Autodesk Inventor part; units mm, degrees
ref_plane "YZ Plane" through (0, 0, 0) normal (1, 0, 0) x (0, 1, 0)
ref_plane "XZ Plane" through (0, 0, 0) normal (0, 1, 0) x (-1, 0, 0)
ref_plane "XY Plane" through (0, 0, 0) normal (0, 0, 1) x (1, 0, 0)
sketch "Sketch7" plane through (0, 0, 0) normal (0, 1, 0) x (-1, 0, 0)
  line L0 (93.98, -93.98) -> (0, -93.98)
  line L1 (0, -87.376) -> (0, -6.604)
  circle A0 centre (101.4857, 19.3548) radius 1.85
  circle A1 centre (101.4857, 19.3548) radius 1.85
  circle A2 centre (-7.5057, 19.3548) radius 1.85
  circle A3 centre (-7.5057, 19.3548) radius 1.85
  circle A4 centre (-7.5057, -113.3348) radius 1.85
  circle A5 centre (101.4857, -113.3348) radius 1.85
  circle A6 centre (101.4857, -113.3348) radius 1.85
  arc A7 (104.7877, 19.3548) -> (98.1837, 19.3548) centre (101.4857, 19.3548) ccw
  arc A8 (-4.2037, 19.3548) -> (-10.8077, 19.3548) centre (-7.5057, 19.3548) ccw
  arc A9 (-10.8077, -113.3348) -> (-4.2037, -113.3348) centre (-7.5057, -113.3348) ccw
  arc A10 (98.1837, -113.3348) -> (104.7877, -113.3348) centre (101.4857, -113.3348) ccw
  line L2 (98.1837, 19.3548) -> (98.1837, 0)
  line L3 (98.1837, 0) -> (93.98, 0)
  line L4 (104.7877, 19.3548) -> (104.7877, 0)
  line L5 (104.7877, 0) -> (104.7877, -6.604)
  line L6 (104.7877, -6.604) -> (93.98, -6.604)
  arc A11 (98.1837, -113.3348) -> (104.7877, -113.3348) centre (101.4857, -113.3348) ccw
  line L7 (98.1837, -113.3348) -> (98.1837, -93.98)
  line L8 (98.1837, -93.98) -> (93.98, -93.98)
  line L9 (104.7877, -113.3348) -> (104.7877, -93.98)
  line L10 (104.7877, -93.98) -> (104.7877, -87.376)
  line L11 (104.7877, -87.376) -> (93.98, -87.376)
  arc A12 (-4.2037, 19.3548) -> (-10.8077, 19.3548) centre (-7.5057, 19.3548) ccw
  line L12 (-4.2037, 19.3548) -> (-4.2037, 0)
  line L13 (-4.2037, 0) -> (0, 0)
  line L14 (-10.8077, 19.3548) -> (-10.8077, 0)
  line L15 (-10.8077, 0) -> (-10.8077, -6.604)
  line L16 (-10.8077, -6.604) -> (0, -6.604)
  arc A13 (-10.8077, -113.3348) -> (-4.2037, -113.3348) centre (-7.5057, -113.3348) ccw
  line L17 (-4.2037, -113.3348) -> (-4.2037, -93.98)
  line L18 (-10.8077, -113.3348) -> (-10.8077, -93.98)
  line L19 (-10.8077, -87.376) -> (0, -87.376)
  line L20 (-4.2037, -93.98) -> (0, -93.98)
  line L21 (-10.8077, -93.98) -> (-10.8077, -87.376)
  circle A14 centre (88.9, -5.08) radius 1.75
  circle A15 centre (88.9, -88.9) radius 1.75
  circle A16 centre (5.08, -5.08) radius 1.75
  circle A17 centre (5.08, -88.9) radius 1.75
  line L22 (98.1837, 0) -> (-4.2037, 0)
  circle A18 centre (80.64, -80.3026) radius 1.75
  circle A19 centre (80.64, -52.1326) radius 1.75
  circle A20 centre (28.58, -85.1226) radius 1.75
  circle A21 centre (29.83, -36.8026) radius 1.75
  circle A22 centre (81.275, -18.8574) radius 1.75
  circle A23 centre (12.705, -18.8574) radius 1.75
  line L23 (88.9, -5.08) -> (90.65, -5.08) construction
  circle A24 centre (111.661, -36.195) radius 2
  circle A25 centre (111.661, -57.785) radius 2
  circle A26 centre (96.421, -36.195) radius 2
  circle A27 centre (96.421, -57.785) radius 2
  line L24 (93.98, -32.484) -> (114.102, -32.484)
  line L25 (114.102, -32.484) -> (115.372, -32.484)
  line L26 (115.372, -32.484) -> (115.372, -60.226)
  line L27 (115.372, -60.226) -> (115.372, -61.496)
  line L28 (115.372, -61.496) -> (93.98, -61.496)
  line L29 (93.98, -61.496) -> (93.98, -87.376)
  line L30 (93.98, -6.604) -> (93.98, -32.484)
  point P0 (-2.54, 0.1)
extrude "Extrusion5" add sketch "Sketch7" along normal blind 1.5875
fillet "Fillet8" radius 6.35 8 edges at (-98.1837, 0.7937, 0) (-93.98, 0.7937, -6.604) (4.2037, 0.7937, 0) (0, 0.7937, -6.604) (0, 0.7937, -87.376) (4.2037, 0.7937, -93.98) (-93.98, 0.7937, -87.376) (-98.1837, 0.7937, -93.98)
fillet "Fillet9" radius 3.175 8 edges at (-104.7877, 0.7937, -6.604) (-115.372, 0.7937, -32.484) (-93.98, 0.7937, -32.484) (-93.98, 0.7937, -61.496) (-115.372, 0.7937, -61.496) (-104.7877, 0.7937, -87.376) (10.8077, 0.7937, -87.376) (10.8077, 0.7937, -6.604)
properties part number "groundPlate"
Geometry check sheet. Reference: the model listing, model coordinates, mm. A direction names the side the tool comes from. Round coordinates to 2 decimals unless told otherwise and drop trailing zeros. Write each loop counter-clockwise with the first axis right and the second up, starting at its lowest first coordinate (ties: lowest second). Pieces come first, ordered by that corner, then holes. Notation, with made-up numbers: (-11.75, 25) -> (20.25, 25) arc R35 cw to (20.25, 57) -> close; hole circle Ø3 at (58.5, 0.25). An arc over 180 degrees is marked (long way). Put each result on its own line as item: value.
1) Thickness scan on probe 1 along Z at (x, y) = (-81, 0.65); probe 2 along Z at (x, y) = (-29.83, 0.85); probe 3 along X at (y, z) = (0.85, 14). Record the ranges inside material, lowest first. Write a range as from..to.
Recorded:
probe 1: z = -93.98..-82.02, -78.59..-53.85, -50.42..-20.59, -17.13..0
probe 2: z = -93.98..-86.35, -83.9..-38.55, -35.05..0
probe 3: x = -104.79..-98.18, 4.2..10.81
2) Cross-section at C-C, the plane z = -5.08. Enter the section's corners in (x, y), plus the area to 3 significant figures.
Recorded:
outline: (-104.32, 0) -> (-90.65, 0) -> (-90.65, 1.59) -> (-104.32, 1.59) -> close; (-87.15, 0) -> (-6.83, 0) -> (-6.83, 1.59) -> (-87.15, 1.59) -> close; (-3.33, 0) -> (10.34, 0) -> (10.34, 1.59) -> (-3.33, 1.59) -> close
area: 171 mm2
3) Cross-section at A-A, the plane z = -108. Enter the section's corners in (x, y).
Recorded:
outline: (-104.79, 0) -> (-98.18, 0) -> (-98.18, 1.59) -> (-104.79, 1.59) -> close; (4.2, 0) -> (10.81, 0) -> (10.81, 1.59) -> (4.2, 1.59) -> close
4) Cross-section at B-B, the plane x = -5.08. Enter the section's corners in (y, z), plus the area to 3 significant figures.
Recorded:
outline: (0, -93.98) -> (1.59, -93.98) -> (1.59, -90.65) -> (0, -90.65) -> close; (0, -87.15) -> (1.59, -87.15) -> (1.59, -6.83) -> (0, -6.83) -> close; (0, -3.33) -> (1.59, -3.33) -> (1.59, 0) -> (0, 0) -> close
area: 138 mm2
5) Cross-section at D-D, the plane z = -45. Enter the section's corners in (x, y).
Recorded:
outline: (-115.37, 0) -> (0, 0) -> (0, 1.59) -> (-115.37, 1.59) -> close
6) Depth check by flat-ended pin: P1, Ø0.8, axis at x = -108.5, y = 0.5, coming from the +Z side; P2, Ø0.8, axis at y = 0.5, z = 10.5, coming from the -X side. Enter the tip coordinate at first touch or a pass-through.
Recorded:
P1: stops at z = -32.48
P2: stops at x = -104.79
7) Access from +Z, -Z, +X, -X, +Y, -Y to the whole of each face (thin tool, end or side, straight path). Record for faces 1 (the face through (9.9, 0.8, -5.65)), 2 (the face through (-95.791, 0.805, -85.466)), 3 (the face through (-109.663, 0.783, -36.283)).
Recorded:
face 1: +X, +Y, -Y
face 2: -X, +Y, -Y
face 3: +Y, -Y
